Autodesk Fusion 360 part; units mm, degrees
sketch "Sketch1" plane through (0, 0, 0) normal (0, 1, 0) x (1, 0, 0) in component "Bottom of Box"
  line L0 (-184.0142, 60) -> (15.9858, 60)
  line L1 (15.9858, 60) -> (15.9858, -40)
  line L2 (15.9858, -40) -> (-184.0142, -40)
  line L3 (-184.0142, -40) -> (-184.0142, 60)
  line L4 (-169.0142, 45) -> (0.9858, 45)
  line L5 (0.9858, 45) -> (0.9858, -25)
  line L6 (0.9858, -25) -> (-169.0142, -25)
  line L7 (-169.0142, -25) -> (-169.0142, 45)
  dimension "d1" = 100
  dimension "d2" = 200
  dimension "d3" = 170
  dimension "d4" = 70
  dimension "d5" = 15
  dimension "d6" = 15
extrude "Extrude1" add sketch "Sketch1" along normal blind 100 contours L0 L1 L2 L3 | L4 L5 L6 L7 in component "Bottom of Box"
extrude "Extrude2" cut sketch "Sketch1" along normal blind 85 contours L4 L5 L6 L7 in component "Bottom of Box"
fillet "Fillet1" radius 10 1 edges at (15.9858, 50, -60) in component "Bottom of Box"
fillet "Fillet2" radius 10 1 edges at (15.9858, 50, 40) in component "Bottom of Box"
fillet "Fillet3" radius 10 1 edges at (-184.0142, 50, 40) in component "Bottom of Box"
fillet "Fillet4" radius 10 1 edges at (-184.0142, 50, -60) in component "Bottom of Box"
sketch "Sketch1 (2)" plane through (0, 0, 0) normal (0, 1, 0) x (1, 0, 0)
  line L0 (-69.0142, -25) -> (-99.0142, -25)
  line L1 (-99.0142, -25) -> (-99.0142, 22)
  line L2 (-99.0142, 22) -> (-69.0142, 22)
  line L3 (-69.0142, 22) -> (-69.0142, -25)
  line L4 (0.9858, -25) -> (0.9858, 45)
  dimension "d30" = 30
  dimension "d31" = 70
  dimension "d79" = 47
extrude "Extrude4" add sketch "Sketch1 (2)" along normal blind 20 in component "Bottom of Box"
sketch "Sketch2" plane through (0, 0, 0) normal (0, 1, 0) x (1, 0, 0)
  circle A0 centre (-84.0142, 7) radius 7.5
  line L0 (-99.0142, 22) -> (-69.0142, 22)
  line L1 (-99.0142, -25) -> (-99.0142, 22)
  dimension "d34" = 15
  dimension "d35" = 15
  dimension "d36" = 15
extrude "Extrude5" add sketch "Sketch2" against normal blind 25 in component "Bottom of Box"
sketch "Sketch3" plane through (0, 0, 0) normal (1, 0, 0) x (0, 0, -1)
  curve A0
  line L0 (-0.5, -25) -> (14.5, -25)
  dimension "d40" = 12.5
  dimension "d81" = 12.5
extrude "Extrude7" cut 1 faces at (-82.4555, -25, -8.9546) along direction (0, 1, 0) blind 10 in component "Bottom of Box"
extrude "Extrude8" add 1 faces at (-82.4555, -15, -8.9546) along direction (0, -1, 0) blind 19 in component "Bottom of Box"
sketch "Sketch5" plane through (0, 0, 0) normal (0, -1, 0) x (1, 0, 0)
  circle A0 centre (-84.0142, -7) radius 7.5
  line L0 (-169.0142, -45) -> (-169.0142, 25)
  line L1 (-169.0142, 25) -> (-99.0142, 25)
  line L2 (-99.0142, 25) -> (-99.0142, -22)
  line L3 (-99.0142, -22) -> (-69.0142, -22)
  line L4 (-69.0142, -22) -> (-69.0142, 25)
  line L5 (-69.0142, 25) -> (0.9858, 25)
  line L6 (0.9858, 25) -> (0.9858, -45)
  line L7 (0.9858, -45) -> (-169.0142, -45)
  arc A1 (-184.0142, -50) -> (-174.0142, -60) centre (-174.0142, -50) ccw
  line L8 (-174.0142, -60) -> (5.9858, -60)
  arc A2 (5.9858, -60) -> (15.9858, -50) centre (5.9858, -50) ccw
  line L9 (15.9858, -50) -> (15.9858, 30)
  arc A3 (15.9858, 30) -> (5.9858, 40) centre (5.9858, 30) ccw
  line L10 (5.9858, 40) -> (-174.0142, 40)
  arc A4 (-174.0142, 40) -> (-184.0142, 30) centre (-174.0142, 30) ccw
  line L11 (-184.0142, 30) -> (-184.0142, -50)
  line L12 (-170.0142, -56) -> (1.9858, -56)
  line L13 (11.9858, -46) -> (11.9858, 26)
  line L14 (1.9858, 36) -> (-170.0142, 36)
  line L15 (-180.0142, 26) -> (-180.0142, -46)
  line L16 (-173.0142, -49) -> (4.9858, -49)
  line L17 (4.9858, -49) -> (4.9858, 29)
  line L18 (4.9858, 29) -> (-173.0142, 29)
  line L19 (-173.0142, 29) -> (-173.0142, -49)
  arc A5 (11.9858, 26) -> (1.9858, 36) centre (1.9858, 26) ccw
  arc A6 (1.9858, -56) -> (11.9858, -46) centre (1.9858, -46) ccw
  arc A7 (-180.0142, -46) -> (-170.0142, -56) centre (-170.0142, -46) ccw
  arc A8 (-170.0142, 36) -> (-180.0142, 26) centre (-170.0142, 26) ccw
  point P0 (-180.0142, -56)
  point P1 (11.9858, -56)
  dimension "d52" = 192
  dimension "d53" = 92
  dimension "d54" = 4
  dimension "d55" = 4
  dimension "d56" = 78
  dimension "d57" = 178
  dimension "d58" = 7
  dimension "d59" = 7
  dimension "d60" = 10
extrude "Extrude10" cut sketch "Sketch5" against normal blind 15 contours L12 L13 L14 L15 A5 A6 A7 A8 in component "Bottom of Box"
sketch "Sketch6" plane through (0, 0, 0) normal (1, 0, 0) x (0, 0, -1)
sketch "Sketch7" plane through (0, 0, 0) normal (1, 0, 0) x (0, 0, -1)
  circle A0 centre (7, -21) radius 5.75
  line L0 (-0.5, -34) -> (14.5, -34)
  dimension "d69" = 7.5
  dimension "d82" = 11.5
  dimension "d84" = 13
extrude "Extrude11" cut sketch "Sketch7" against normal blind 100 in component "Bottom of Box"
component "Bottom of Box" placed x (1, 0, 0) y (0, 1, 0) z (0, 0, 1) at (0, 0, 0)
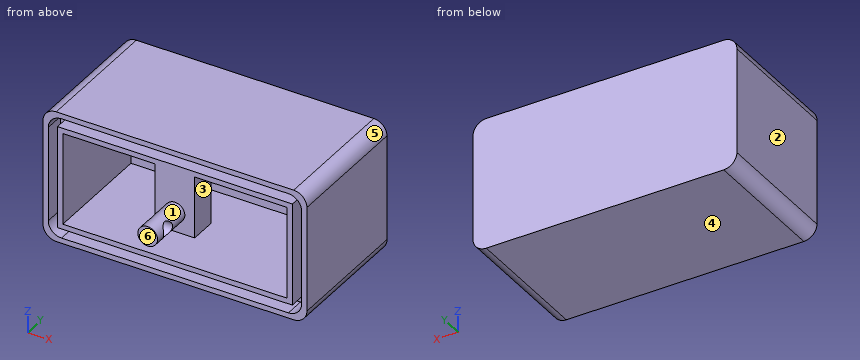
The listing builds one solid part. Answer for the finished solid, in the listing's coordinates (mm). Face numbers are marked on the shaded views. A direction names the side the tool comes from. Round coordinates to 2 decimals unless told otherwise and drop trailing zeros. Loops run counter-clockwise (first coordinate to the right, second up) from the corner with the lowest first, then second, coordinate; pieces in that order, holes last. Notation, with made-up numbers: (-39, 72.5) - (7, 72.5) arc R16 ccw to (7, 92.5) - close; hole circle Ø3 at (53.25, -31.5). An arc over 180 degrees is marked (long way). Use one line per item in the form item = value. Start each with the question number.
1. The part is cut by section B-B on y = 17.5. Determine the outline of the cut face in (x, z), then the cut area to 3 significant figures.
2. The part is cut by section A-A on z = -7. Determine the outline of the cut face in (x, y), then the cut area to 3 significant figures.
3. Given pin 1 Ø5 at (y, z) = (-17, 2) entering from +X, flat-ended and moving along its own axis, determine where the tip first touches the part or whether it passes through.
4. The part is cut by section C-C on z = -39.5. Determine the outline of the cut face in (x, y).
5. A tool of negligible diameter and unlimited length cuts with its end or side. For the marked faces 1 and 2, from which of +Z, -Z, +X, -X, +Y, -Y can it reach the whole face along a straight path? Write none if from no direction.
6. The part is cut by section D-D on x = -18.5. Determine the outline of the cut face in (y, z).
7. For a pull along Z with two mould halves and no side action, classify the marked faces 3, 4, 5 and 6 as pulls with the +Z half, pulls with the -Z half, needs draft (parallel to the pull), parting line crosses it, or undercut.
8. Consider line 1 (Z direction, x = -87, y = 8); line 2 (Y direction, x = -87, z = -7); line 3 (X direction, y = 70, z = -16.5). Determine where each line is inside the solid, lowest interval first. Write a range as [from, to].
Geometry check:
q1.outline = (-184.01, -50) arc R10 ccw to (-174.01, -60) - (5.99, -60) arc R10 ccw to (15.99, -50) - (15.99, 30) arc R10 ccw to (5.99, 40) - (-174.01, 40) arc R10 ccw to (-184.01, 30) - close; hole (-169.01, -45) - (0.99, -45) - (0.99, 25) - (-69.01, 25) - (-69.01, -22) - (-99.01, -22) - (-99.01, 25) - (-169.01, 25) - close
q1.area = 9,420 mm^2
q2.outline = (-184.01, 0) - (-180.01, 0) - (-180.01, 15) - (-173.01, 15) - (-173.01, 0) - (-169.01, 0) - (-169.01, 85) - (0.99, 85) - (0.99, 0) - (4.99, 0) - (4.99, 15) - (11.99, 15) - (11.99, 0) - (15.99, 0) - (15.99, 100) - (-184.01, 100) - close; (-99.01, 0) - (-91.51, 0) - (-91.51, -15.25) - (-76.51, -15.25) - (-76.51, 0) - (-69.01, 0) - (-69.01, 20) - (-99.01, 20) - close; (-91.51, -34) - (-76.51, -34) - (-76.51, -26.75) - (-91.51, -26.75) - close
q2.area = 6,280 mm^2
q3.pin_1 = -80.27
q4.outline = (-184.01, 0) - (-180.01, 0) - (-180.01, 15) - (-173.01, 15) - (-173.01, 0) - (-169.01, 0) - (-169.01, 85) - (0.99, 85) - (0.99, 0) - (4.99, 0) - (4.99, 15) - (11.99, 15) - (11.99, 0) - (15.99, 0) - (15.99, 100) - (-184.01, 100) - close
q5.face_1 = -Y
q5.face_2 = +Z, -Z, -X, +Y, -Y
q6.outline = (0, -60) - (100, -60) - (100, 40) - (0, 40) - (0, 36) - (15, 36) - (15, 29) - (0, 29) - (0, 25) - (85, 25) - (85, -45) - (0, -45) - (0, -49) - (15, -49) - (15, -56) - (0, -56) - close
q7.face_3 = undercut
q7.face_4 = pulls with the -Z half
q7.face_5 = pulls with the +Z half
q7.face_6 = needs draft
q8.line_1 = [-60, -56], [-49, -45], [-22, 29], [36, 40]
q8.line_2 = [-34, -26.75], [-15.25, 20], [85, 100]
q8.line_3 = [-184.01, -169.01], [0.99, 15.99]
